from build123d import *

# Parameters (mm, degrees)
REVOLVE_THIN1_OUTLINE_W   = 10
REVOLVE_THIN1_OUTLINE_H   = 4.190294711
REVOLVE_THIN1_OUTLINE_H_2 = 25.430398101
SKETCH4_W                 = 50.454885555
SKETCH4_H                 = 34.702925128
BOSS_EXTRUDE1_DEPTH       = 25
SKETCH5_R                 = 6.92656428
CUT_EXTRUDE1_DEPTH        = 50


# Read off the part's stored shape, not the designer's step: Revolve-Thin1
with BuildPart() as part:
    # Revolve-Thin1 outline → Revolve-Thin1 (revolve)
    with BuildSketch(Plane.XY):
        with BuildLine():
            Line((12.572695835, -4.190294711), (2.572695835, -4.190294711))
            add(Edge.make_bspline(
                [(2.572695835, -4.190294711), (3.256803477, -4.863264231), (4.111938029, -5.704476131), (5.052586036, -6.629809221), (5.351883129, -6.924233386), (5.480153312, -7.050415171), (5.565666767, -7.134536361), (5.60649606, -7.174703671), (5.975784665, -7.538349261), (7.610779142, -9.157595772), (9.214355978, -10.792063367), (11.18191941, -12.844557715), (11.880423743, -13.582762852), (12.572695835, -14.324008024)],
                knots=[0, 0, 0, 0, 0.015625, 0.01953125, 0.021484375, 0.022460937, 0.022460937, 0.0234375, 0.0234375, 0.03125, 0.0625, 0.0625, 0.079939883, 0.079939883, 0.079939883, 0.079939883], degree=3))
            Line((12.572695835, -14.324008024), (12.572695835, -4.190294711))
        make_face()
        with Locations((7.572695835, -2.095147355)):
            Rectangle(REVOLVE_THIN1_OUTLINE_W, REVOLVE_THIN1_OUTLINE_H)
        with BuildLine():
            Line((12.572695835, -4.190294711), (12.572695835, -14.324008024))
            add(Edge.make_bspline(
                [(12.572695835, -14.324008024), (14.361346695, -16.239192574), (16.108392925, -18.174671527), (22.545566832, -25.556112446), (26.95842293, -31.138237836), (39.252867809, -48.361072942), (46.191672462, -60.477354516), (57.598611585, -86.045280246), (62.066987666, -99.498416997), (68.499575811, -127.673184033), (70.487892964, -142.381255893), (71.247958055, -157.804064752)],
                knots=[0.079939883, 0.079939883, 0.079939883, 0.079939883, 0.125, 0.125, 0.25, 0.25, 0.5, 0.5, 0.75, 0.75, 0.997458266, 0.997458266, 0.997458266, 0.997458266], degree=3))
            Line((71.247958055, -157.804064752), (71.270990011, -157.804064752))
            Line((71.270990011, -157.804064752), (71.270990011, -96.986600276))
            add(Edge.make_bspline(
                [(16.732968649, -4.190294711), (55.715421715, -44.398968265), (71.270990011, -96.986600276)],
                knots=[0.032914248, 0.032914248, 0.032914248, 0.659474661, 0.659474661, 0.659474661], degree=2))
            Line((16.732968649, -4.190294711), (12.572695835, -4.190294711))
        make_face()
        with Locations((7.572695835, 12.715199051)):
            Rectangle(REVOLVE_THIN1_OUTLINE_W, REVOLVE_THIN1_OUTLINE_H_2)
        with BuildLine():
            Line((12.572695835, 0), (12.572695835, -4.190294711))
            Line((12.572695835, -4.190294711), (16.732968649, -4.190294711))
            add(Edge.make_bspline(
                [(12.572695835, 0), (14.685156347, -2.078067033), (16.732968649, -4.190294711)],
                knots=[0, 0, 0, 0.032914248, 0.032914248, 0.032914248], degree=2))
        make_face()
        with BuildLine():
            Line((71.270990011, -157.804064752), (71.247958055, -157.804064752))
            add(Edge.make_bspline(
                [(71.247958055, -157.804064752), (71.255764961, -157.96247806), (71.263442286, -158.120966773), (71.270990011, -158.279530915)],
                knots=[0.997458266, 0.997458266, 0.997458266, 0.997458266, 1, 1, 1, 1], degree=3))
            Line((71.270990011, -158.279530915), (71.270990011, -157.804064752))
        make_face()
        Polygon((71.270990011, -157.804064752), (71.270990011, -158.279530915), (81.259680211, -157.804064752), align=None)
        with BuildLine():
            Line((71.270990011, -96.986600276), (71.270990011, -157.804064752))
            Line((71.270990011, -157.804064752), (81.259680211, -157.804064752))
            add(Edge.make_bspline(
                [(71.270990011, -96.986600276), (79.725187008, -125.567118335), (81.259680211, -157.804064752)],
                knots=[0.659474661, 0.659474661, 0.659474661, 1, 1, 1], degree=2))
        make_face()
    revolve(axis=Axis((0, 0, 0), (0, 1, 0)))

    # Sketch4 → Boss-Extrude1 (add, symmetric)
    with BuildSketch(Plane.XY):
        with Locations((0.507285531, 17.351462564)):
            Rectangle(SKETCH4_W, SKETCH4_H)
    extrude(amount=BOSS_EXTRUDE1_DEPTH, both=True)

    # Sketch5 → Cut-Extrude1 (cut)
    with BuildSketch(Plane(origin=(0, 34.702925128, 0), x_dir=(1, 0, 0), z_dir=(0, 1, 0))):
        with Locations(Location((0, 0, 0), (0, 0, 270))):
            Circle(SKETCH5_R)
    extrude(amount=-CUT_EXTRUDE1_DEPTH, mode=Mode.SUBTRACT)


solid = part.part
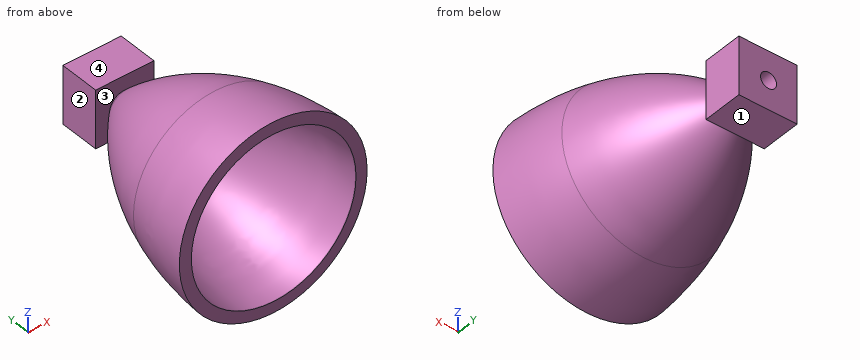
Geometry check sheet. Reference: the model listing, model coordinates, mm. Face numbers are marked on the shaded views. A direction names the side the tool comes from. Round coordinates to 2 decimals unless told otherwise and drop trailing zeros. One line per item, written item: value. Start each with the question number.
(1) Scan lines: line 1 (X direction, y = 19, z = 0); line 2 (Z direction, x = 0, y = 5.5); line 3 (X direction, y = -39, z = -13). Record each from-to range of solid material in increasing order. Write a range as [from, to].
(2) Access from +Z, -Z, +X, -X, +Y, -Y to the whole of each face (thin tool, end or side, straight path). Record for the marked faces 1, 2, 3 and 4.
(3) Go/stop test with flat-tipped pins: pin 1 Ø6 at (x, y) = (-64, -112) entering from +Z; pin 2 Ø1 at (y, z) = (-23.5, -1) entering from -X; pin 3 Ø1 at (y, z) = (-85.5, -22.5) entering from +X; pin 4 Ø12.5 at (x, z) = (0, 0) entering from -Y. Record where each tip stops, or that it passes through.
Answer:
1. line 1: [-24.72, -6.93], [6.93, 25.73]
1. line 2: [-25, -6.93], [6.93, 25]
1. line 3: [-42.67, -29.84], [29.84, 42.67]
2. face 1: -Z, +X, -X, +Y
2. face 2: +Z, -Z, -X, +Y
2. face 3: none
2. face 4: +Z, +X, -X, +Y
3. pin 1: z = 44.1
3. pin 2: x = -33.92
3. pin 3: x = 63.94
3. pin 4: through
